```python
from build123d import *

# Parameters (mm, degrees)
F0_W     = 65
F0_H     = 65
F1_DEPTH = 6
F2_SIZE  = 2
F4_DEPTH = 100


with BuildPart() as f1:
    # F0 (on Top) → F1 (new body)
    with BuildSketch(Plane.XY):
        Rectangle(F0_W, F0_H)
    extrude(amount=F1_DEPTH)

    # F2
    f2_edges = [f1.edges().sort_by_distance(p)[0] for p in [
        (0, -32.5, 6),
        (32.5, 0, 6),
        (0, 32.5, 6),
        (-32.5, 0, 6),
    ]]
    chamfer(f2_edges, length=F2_SIZE)

    # F3 (on face) → F4 (join)
    with BuildSketch(Plane.XY.offset(6)):
        Polygon((27.5, -26.5), (29.5, -28.5), (29.5, 29.5), (-29.5, 29.5), (-29.5, -28.5), (-27.5, -26.5), (-27.5, 27.5), (27.5, 27.5), align=None)
    extrude(amount=F4_DEPTH)


solid = f1.part
```
Here's how the part is built. I have some questions about the finished solid (model axes, mm). A direction names the side the tool comes from. Round coordinates to 2 decimals unless told otherwise and drop trailing zeros. Write each loop counter-clockwise with the first axis right and the second up, starting at its lowest first coordinate (ties: lowest second). Pieces come first, ordered by that corner, then holes.
Q1. If we section it at A-A on y = 2.5: Write out the boundary of the cut face in (x, z), plus the area to 3 significant figures.
Q2. Please list where these lines run through material, in increasing order: probe 1 along X at (y, z) = (23, 38.5); probe 2 along Z at (x, y) = (-15.5, 10); probe 3 along Y at (x, z) = (-16.5, 93.5).
Q3. Will these pins go through, and if not, where does the flat tip stop? P1, Ø10, axis at x = 3.5, z = 50, coming from the -Y side; P2, Ø6, axis at y = 17.5, z = 66, coming from the +X side; P3, Ø1, axis at x = 10, z = 51, coming from the +Y side.
Q4. If we mould it in two halves opening along X, with no side actions, what happens to faces 1 (the flat face through (27.5, 1, 55)), 2 (the flat face through (29.5, 0, 55)), 3 (the flat face through (0, 29.5, 55))? For each: +X half, -X half, draft (parallel to the pull), parting line (faces both ways), or undercut.
Q5. If we section it at C-C on z = 84.5: Write out the boundary of the cut face in (x, y).
Q6. Which directions (+Z, -Z, +X, -X, +Y, -Y) give clear straight access to the entire face, cutting with the end or side of a thin tool? Please do faces 4 (the flat face through (-32.5, 0, 2)), 5 (the flat face through (0, 27.5, 55)), 6 (the flat face through (-29.5, 1, 55)).
Q7. If we section it at B-B on x = -4: Write out the boundary of the cut face in (y, z).
Answer below:
1. outline: (-32.5, 0) - (32.5, 0) - (32.5, 4) - (30.5, 6) - (29.5, 6) - (29.5, 106) - (27.5, 106) - (27.5, 6) - (-27.5, 6) - (-27.5, 106) - (-29.5, 106) - (-29.5, 6) - (-30.5, 6) - (-32.5, 4) - close
1. area: 786 mm2
2. probe 1: x = -29.5 to -27.5, 27.5 to 29.5
2. probe 2: z = 0 to 6
2. probe 3: y = 27.5 to 29.5
3. P1: stops at y = 27.5
3. P2: stops at x = 29.5
3. P3: stops at y = 29.5
4. face 1: undercut
4. face 2: +X half
4. face 3: draft
5. outline: (-29.5, -28.5) - (-27.5, -26.5) - (-27.5, 27.5) - (27.5, 27.5) - (27.5, -26.5) - (29.5, -28.5) - (29.5, 29.5) - (-29.5, 29.5) - close
6. face 4: +Z, -Z, -X, +Y, -Y
6. face 5: +Z, -Y
6. face 6: +Z, -X, +Y, -Y
7. outline: (-32.5, 0) - (32.5, 0) - (32.5, 4) - (30.5, 6) - (29.5, 6) - (29.5, 106) - (27.5, 106) - (27.5, 6) - (-30.5, 6) - (-32.5, 4) - close
